The figure shows three views and two pictorial views of one solid part (mm, origin at its lowest corner). Answer the questions. Coordinates: 2 decimals unless noted, no trailing zeros. Loops run counter-clockwise (first coordinate to the right, second up) from the corner with the lowest first, then second, coordinate; pieces in that order, holes last.
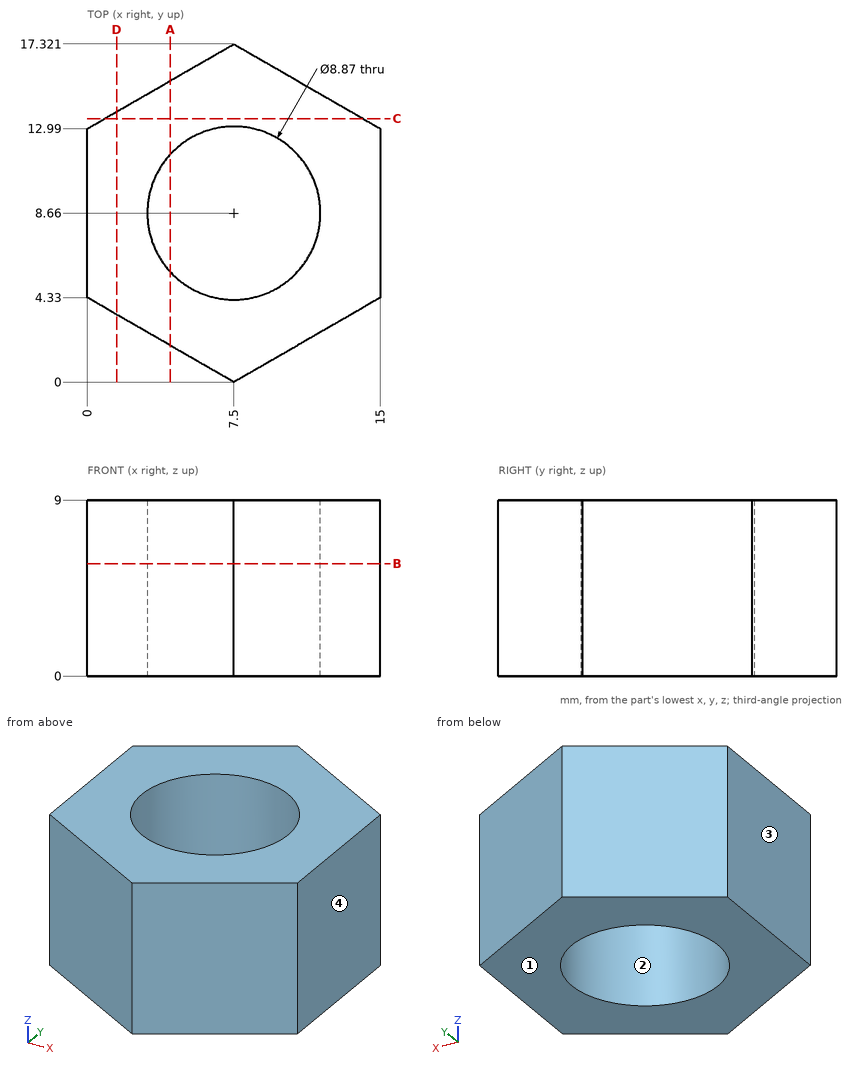
1. A cutting plane is placed at B-B, the plane z = 5.75. Give the vertices of the cut face in (x, y) (1 decimal), then the cut area to 3 significant figures.
2. Determine the mould class of the marked faces 1, 2, 3 and 4 for opening direction X: released by +X, released by -X, zero draft, split by the parting line, or undercut.
3. A cutting plane is placed at D-D, the plane x = 1.5. Give the vertices of the cut face in (y, z).
4. Straight lines are drawn through the part: probe 1 along X at (y, z) = (6, 4); probe 2 along Y at (x, z) = (5.5, 7.25) (1 decimal); probe 3 along Y at (x, z) = (6.75, 0.75). For each, find the intervals that lie inside material, in ascending order.
5. A cutting plane is placed at A-A, the plane x = 4.25. Give the vertices of the cut face in (y, z).
6. Each of these flat-tipped pins is pushed along its axis until it touches: P1, Ø1.5, axis at x = 2, z = 6.5, coming from the +Y side; P2, Ø7, axis at x = 7.5, y = 8.66, coming from the +Z side; P3, Ø1.5, axis at y = 2.5, z = 1, coming from the -X side; P4, Ø2, axis at y = 3.5, z = 4, coming from the -X side. Where does it stop, or does it pass through?
7. A cutting plane is placed at C-C, the plane y = 13.5. Give the vertices of the cut face in (x, z), then the cut area to 3 significant figures.
Answers below:
1. outline: (0, 4.3) - (7.5, 0) - (15, 4.3) - (15, 13) - (7.5, 17.3) - (0, 13) - close; hole circle Ø8.9 at (7.5, 8.7)
1. area: 133 mm2
2. face 1: zero draft
2. face 2: undercut
2. face 3: released by -X
2. face 4: released by +X
3. outline: (3.46, 0) - (13.86, 0) - (13.86, 9) - (3.46, 9) - close
4. probe 1: x = 0 to 3.95, 11.05 to 15
4. probe 2: y = 1.2 to 4.7, 12.6 to 16.2
4. probe 3: y = 0.43 to 4.29, 13.03 to 16.89
5. outline: (1.88, 0) - (5.64, 0) - (5.64, 9) - (1.88, 9) - close; (11.68, 0) - (15.44, 0) - (15.44, 9) - (11.68, 9) - close
6. P1: stops at y = 14.58
6. P2: passes through
6. P3: stops at x = 1.87
6. P4: stops at x = 0
7. outline: (0.88, 0) - (14.12, 0) - (14.12, 9) - (0.88, 9) - close
7. area: 119 mm2
